from build123d import *

# Parameters (mm, degrees)
SKETCH_1_W          = 48
SKETCH_1_H          = 47
SKETCH_1_R          = 14
EXTRUDE_1_DEPTH     = 63
SKETCH_2_R          = 2.5
CUT_EXTRUDE_1_DEPTH = 49
SKETCH_3_R          = 2.75
CUT_EXTRUDE_2_DEPTH = 10


with BuildPart() as part:
    # Эскиз1 → Бобышка-Вытянуть1 (new body)
    with BuildSketch(Plane(origin=(0, 0, 0), x_dir=(1, 0, 0), z_dir=(0, 1, 0))):
        Rectangle(SKETCH_1_W, SKETCH_1_H)
        Circle(SKETCH_1_R, mode=Mode.SUBTRACT)
    extrude(amount=EXTRUDE_1_DEPTH)

    # Эскиз2 → Вырез-Вытянуть1 (cut, through all)
    with BuildSketch(Plane.ZY.offset(24)):
        with Locations((-19.000000006, 47.3)):
            Circle(SKETCH_2_R)
        with Locations((-19.000000006, 17.3)):
            Circle(SKETCH_2_R)
        with Locations((18.999999994, 47.3)):
            Circle(SKETCH_2_R)
        with Locations((18.999999994, 17.3)):
            Circle(SKETCH_2_R)
    extrude(amount=-CUT_EXTRUDE_1_DEPTH, mode=Mode.SUBTRACT)

    # Эскиз3 → Вырез-Вытянуть2 (cut)
    with BuildSketch(Plane(origin=(0, 63, 0), x_dir=(1, 0, 0), z_dir=(0, 1, 0))):
        with Locations((13.435028843, -13.435028842)):
            Circle(SKETCH_3_R)
        with Locations((0, -19)):
            Circle(SKETCH_3_R)
        with Locations((-13.435028842, -13.435028842)):
            Circle(SKETCH_3_R)
        with Locations((13.435028843, 13.435028843)):
            Circle(SKETCH_3_R)
        with Locations((0, 19)):
            Circle(SKETCH_3_R)
        with Locations((-13.435028842, 13.435028843)):
            Circle(SKETCH_3_R)
    extrude(amount=-CUT_EXTRUDE_2_DEPTH, mode=Mode.SUBTRACT)


solid = part.part
Can you work these out from the model? Positions are in its coordinate system, mm. A direction names the side the tool comes from. Give positions to 0.01 mm unless a question says otherwise; leave off trailing zeros. Order: outer loops, then holes, each group sorted by start corner. A loop starts at its lowest first (then second) coordinate and runs counter-clockwise, first axis right, second up. Notation, with made-up numbers: M -2,-5 L 22,-5 A27 ccw 22,32 Z; hole C -9,-20.5 d10. An arc over 180 degrees is marked long. Use one line per item in the form item = value.
Item 1: If we section it at C-C, the plane z = 0: Write out the boundary of the cut face in (x, y), and give its area (3 significant figures).
Values follow:
outline = M -24,0 L -14,0 L -14,63 L -24,63 Z; M 14,0 L 24,0 L 24,63 L 14,63 Z
area = 1,260 mm^2
Item 2: Will this pin go through, and if not, where does the flat tip stop? pin 1 Ø1.6 at (x, z) = (14, 12.5) entering from +Y.
Values follow:
pin_1 = 53
Item 3: Thinking about a two-plate mould opening in Y: for faces 1 (the cylindrical face through (-11.957, 58.07, 11.116)), 2 (the cylindrical face through (-0.34, 49.41, 20.34)), 3 (the cylindrical face through (-0.34, 49.41, -17.66)), 4 (the flat face through (-13, 53, -13)), which applies, pulls with the +Y half, pulls with the -Y half, needs draft (parallel to the pull), parting line crosses it, or undercut?
Values follow:
face_1 = needs draft
face_2 = undercut
face_3 = undercut
face_4 = pulls with the +Y half
Item 4: If I drill on line 1 along Z through (x, y) = (0, 60.5); line 2 along Y through (x, z) = (-1, 19); line 3 along X through (y, z) = (56, 19), over which ranges is the centre line in solid material (lowest first)? Write a range as [from, to].
Values follow:
line_1 = [-23.5, -21.75], [-16.25, -14], [14, 16.25], [21.75, 23.5]
line_2 = [0, 14.8], [19.8, 44.8], [49.8, 53]
line_3 = [-24, -2.75], [2.75, 24]
Item 5: If we section it at D-D, the plane z = -19: Write out the boundary of the cut face in (x, y).
Values follow:
outline = M -24,0 L 24,0 L 24,14.8 L -24,14.8 Z; M -24,19.8 L 24,19.8 L 24,44.8 L -24,44.8 Z; M -24,49.8 L 24,49.8 L 24,63 L 2.75,63 L 2.75,53 L -2.75,53 L -2.75,63 L -24,63 Z
Item 6: For faces 5 (the flat face through (10, 0, -11)), 6 (the flat face through (0, 53, 19)), which set-ups out of +Z, -Z, +X, -X, +Y, -Y let a thin tool reach every point of the face, with its end or its side?
Values follow:
face_5 = +Z, -Z, +X, -X, -Y
face_6 = +Y
Item 7: If we section it at A-A, the plane x = 0: Write out the boundary of the cut face in (y, z), and give its area (3 significant figures).
Values follow:
outline = M 0,-23.5 L 63,-23.5 L 63,-21.75 L 53,-21.75 L 53,-16.25 L 63,-16.25 L 63,-14 L 0,-14 Z; M 0,14 L 63,14 L 63,16.25 L 53,16.25 L 53,21.75 L 63,21.75 L 63,23.5 L 0,23.5 Z; hole C 17.3,-19 d5; hole C 17.3,19 d5; hole C 47.3,-19 d5; hole C 47.3,19 d5
area = 1,010 mm^2
Item 8: If we section it at B-B, the plane y = 17.3: Write out the boundary of the cut face in (x, z), and give its area (3 significant figures).
Values follow:
outline = M -24,-23.5 L 24,-23.5 L 24,-21.5 L -24,-21.5 Z; M -24,-16.5 L 24,-16.5 L 24,16.5 L -24,16.5 Z; M -24,21.5 L 24,21.5 L 24,23.5 L -24,23.5 Z; hole C 0,0 d28
area = 1,160 mm^2
